Can you work these out from the model? Positions are in its coordinate system, mm. Face numbers are marked on the shaded views. Round coordinates to 2 decimals unless told otherwise and drop trailing zeros. Loops run counter-clockwise (first coordinate to the right, second up) from the corner with the lowest first, then second, coordinate; pieces in that order, holes last.
(1) I want a section at C-C on x = 3.7. Write out the boundary of the cut face in (y, z), plus the area to 3 significant figures.
(2) Thinking about a two-plate mould opening in Y: for the marked faces 1, 2 and 3, which applies, released by +Y, released by -Y, zero draft, split by the parting line, or undercut?
(3) I want a section at A-A on y = 0. Write out the boundary of the cut face in (x, z), plus the area to 3 significant figures.
(4) If I drill on line 1 along Z through (x, y) = (2.95, 0); line 2 along Y through (x, z) = (0.6, 0.95); line 3 along Z through (x, y) = (3.55, -0.75), over which ranges is the centre line in solid material (lowest first)?
(5) Will these pins go through, and if not, where does the flat tip stop? pin 1 Ø1 at (x, z) = (2.5, 1) entering from -Y; pin 2 Ø1 at (x, y) = (2, 1) entering from +Z; pin 3 Ø3 at (y, z) = (1, -0.5) entering from +X.
(6) I want a section at D-D on x = 2.15. Write out the boundary of the cut face in (y, z), plus the area to 3 significant figures.
Autodesk Inventor part; units mm, degrees
ref_plane "ip_st_ir_1_1_XY" through (2, 3.25, 0) normal (1, 0, 0) x (0, 0, -1)
ref_plane "ip_st_ir_1_1_YZ" through (2, 3.25, 0) normal (0, 0, -1) x (0, 1, 0)
ref_plane "ip_st_ir_1_1_ZX" through (2, 3.25, 0) normal (0, 1, 0) x (1, 0, 0)
sketch "Sketch_1" plane through (0, 0, 0) normal (0, 0, 1) x (1, 0, 0)
  line L0 (4, 0) -> (0, 0)
  arc A0 (0, 2.15) -> (0.15, 2) centre (0.15, 2.15) ccw
  line L1 (0.15, 2) -> (3.85, 2)
  arc A1 (3.85, 2) -> (4, 2.15) centre (3.85, 2.15) ccw
  line L2 (4, 2.15) -> (4, 2.6)
  line L3 (4, 2.6) -> (2.3742, 2.6)
  arc A2 (1.6258, 2.6) -> (2.3742, 2.6) centre (2, 3.25) ccw
  line L4 (1.6258, 2.6) -> (0, 2.6)
  line L5 (0, 2.6) -> (0, 2.15)
revolve "Revolution1" add sketch "Sketch_1" angle 360 about axis through (4, 0, 0) along (1, 0, 0)
ref_plane "ip_st_ir_1_1_XY" through (2, 3.25, 0) normal (1, 0, 0) x (0, 0, -1)
ref_plane "ip_st_ir_1_1_YZ" through (2, 3.25, 0) normal (0, 0, -1) x (0, 1, 0)
ref_plane "ip_st_ir_1_1_ZX" through (2, 3.25, 0) normal (0, 1, 0) x (1, 0, 0)
ref_plane "ip_st_ir_1_10_XY" through (2, 2.6293, -1.9103) normal (1, 0, 0) x (0, 0, -1)
ref_plane "ip_st_ir_1_10_YZ" through (2, 2.6293, -1.9103) normal (0, 0, -1) x (0, 1, 0)
ref_plane "ip_st_ir_1_10_ZX" through (2, 2.6293, -1.9103) normal (0, 1, 0) x (1, 0, 0)
ref_plane "ip_st_ir_1_2_XY" through (2, 2.6293, 1.9103) normal (1, 0, 0) x (0, 0, -1)
ref_plane "ip_st_ir_1_2_YZ" through (2, 2.6293, 1.9103) normal (0, 0, -1) x (0, 1, 0)
ref_plane "ip_st_ir_1_2_ZX" through (2, 2.6293, 1.9103) normal (0, 1, 0) x (1, 0, 0)
ref_plane "ip_st_ir_1_3_XY" through (2, 1.0043, 3.0909) normal (1, 0, 0) x (0, 0, -1)
ref_plane "ip_st_ir_1_3_YZ" through (2, 1.0043, 3.0909) normal (0, 0, -1) x (0, 1, 0)
ref_plane "ip_st_ir_1_3_ZX" through (2, 1.0043, 3.0909) normal (0, 1, 0) x (1, 0, 0)
ref_plane "ip_st_ir_1_4_XY" through (2, -1.0043, 3.0909) normal (1, 0, 0) x (0, 0, -1)
ref_plane "ip_st_ir_1_4_YZ" through (2, -1.0043, 3.0909) normal (0, 0, -1) x (0, 1, 0)
ref_plane "ip_st_ir_1_4_ZX" through (2, -1.0043, 3.0909) normal (0, 1, 0) x (1, 0, 0)
ref_plane "ip_st_ir_1_5_XY" through (2, -2.6293, 1.9103) normal (1, 0, 0) x (0, 0, -1)
ref_plane "ip_st_ir_1_5_YZ" through (2, -2.6293, 1.9103) normal (0, 0, -1) x (0, 1, 0)
ref_plane "ip_st_ir_1_5_ZX" through (2, -2.6293, 1.9103) normal (0, 1, 0) x (1, 0, 0)
ref_plane "ip_st_ir_1_6_XY" through (2, -3.25, 0) normal (1, 0, 0) x (0, 0, -1)
ref_plane "ip_st_ir_1_6_YZ" through (2, -3.25, 0) normal (0, 0, -1) x (0, 1, 0)
ref_plane "ip_st_ir_1_6_ZX" through (2, -3.25, 0) normal (0, 1, 0) x (1, 0, 0)
ref_plane "ip_st_ir_1_7_XY" through (2, -2.6293, -1.9103) normal (1, 0, 0) x (0, 0, -1)
ref_plane "ip_st_ir_1_7_YZ" through (2, -2.6293, -1.9103) normal (0, 0, -1) x (0, 1, 0)
ref_plane "ip_st_ir_1_7_ZX" through (2, -2.6293, -1.9103) normal (0, 1, 0) x (1, 0, 0)
ref_plane "ip_st_ir_1_8_XY" through (2, -1.0043, -3.0909) normal (1, 0, 0) x (0, 0, -1)
ref_plane "ip_st_ir_1_8_YZ" through (2, -1.0043, -3.0909) normal (0, 0, -1) x (0, 1, 0)
ref_plane "ip_st_ir_1_8_ZX" through (2, -1.0043, -3.0909) normal (0, 1, 0) x (1, 0, 0)
ref_plane "ip_st_ir_1_9_XY" through (2, 1.0043, -3.0909) normal (1, 0, 0) x (0, 0, -1)
ref_plane "ip_st_ir_1_9_YZ" through (2, 1.0043, -3.0909) normal (0, 0, -1) x (0, 1, 0)
ref_plane "ip_st_ir_1_9_ZX" through (2, 1.0043, -3.0909) normal (0, 1, 0) x (1, 0, 0)
ref_plane "ip_st_ir_1a_XY" through (0, 0, 0) normal (1, 0, 0) x (0, 0, -1)
ref_plane "ip_st_ir_1a_YZ" through (0, 0, 0) normal (0, 0, -1) x (0, 1, 0)
ref_plane "ip_st_ir_1a_ZX" through (0, 0, 0) normal (0, 1, 0) x (1, 0, 0)
ref_plane "ip_st_ir_2a_XY" through (0.2656, 0, 0) normal (1, 0, 0) x (0, 0, -1)
ref_plane "ip_st_ir_2a_YZ" through (0.2656, 0, 0) normal (0, 0, -1) x (0, 1, 0)
ref_plane "ip_st_ir_2a_ZX" through (0.2656, 0, 0) normal (0, 1, 0) x (1, 0, 0)
properties part number "684AZZ Inner Ring"
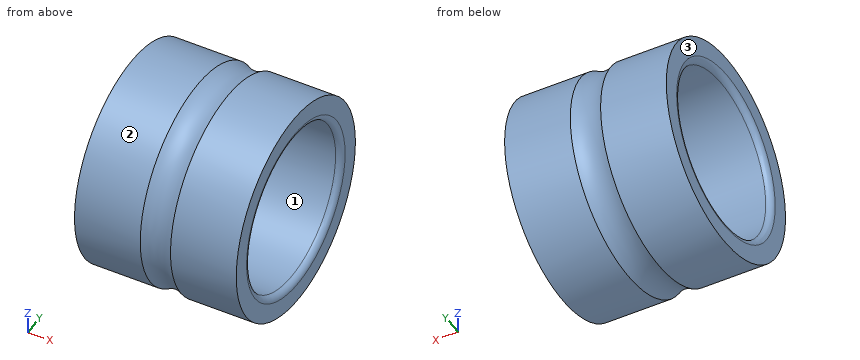
Filled sheet:
1. outline: circle Ø5.2 at (0, 0); hole circle Ø4 at (0, 0)
1. area: 8.67 mm2
2. face 1: undercut
2. face 2: split by the parting line
2. face 3: zero draft
3. outline: (0, -2.6) - (1.63, -2.6) arc R0.75 cw to (2.37, -2.6) - (4, -2.6) - (4, -2.15) arc R0.15 ccw to (3.85, -2) - (0.15, -2) arc R0.15 ccw to (0, -2.15) - close; (0, 2.15) arc R0.15 ccw to (0.15, 2) - (3.85, 2) arc R0.15 ccw to (4, 2.15) - (4, 2.6) - (2.37, 2.6) arc R0.75 cw to (1.63, 2.6) - (0, 2.6) - close
3. area: 4.68 mm2
4. line 1: z = -2.6 to -2, 2 to 2.6
4. line 2: y = -2.42 to -1.76, 1.76 to 2.42
4. line 3: z = -2.49 to -1.85, 1.85 to 2.49
5. pin 1: stops at y = -2.55
5. pin 2: stops at z = 2.51
5. pin 3: stops at x = 4
6. outline: circle Ø5.03 at (0, 0); hole circle Ø4 at (0, 0)
6. area: 7.31 mm2
